Autodesk Inventor part; units mm, degrees
ref_plane "YZ Plane" through (0, 0, 0) normal (1, 0, 0) x (0, 1, 0)
ref_plane "XZ Plane" through (0, 0, 0) normal (0, 1, 0) x (-1, 0, 0)
ref_plane "XY Plane" through (0, 0, 0) normal (0, 0, 1) x (1, 0, 0)
sketch "Эскиз1" plane through (0, 0, 0) normal (0, 1, 0) x (-1, 0, 0)
  line L0 (8.9, -8.9) -> (-8.9, -8.9)
  line L1 (-8.9, -8.9) -> (-8.9, -2.1)
  line L2 (-8.9, 8.9) -> (8.9, 8.9)
  line L3 (8.9, 8.9) -> (8.9, 2.1)
  line L4 (0, 0) -> (0, -10.3494) construction
  line L5 (0, 0) -> (-17.6402, 0) construction
  circle A0 centre (10, 0) radius 0.9 construction
  circle A1 centre (-10, 0) radius 0.9 construction
  arc A2 (10, -2.1) -> (10, 2.1) centre (10, 0) ccw
  line L6 (10, -2.1) -> (8.9, -2.1)
  line L7 (10, 2.1) -> (8.9, 2.1)
  line L8 (8.9, -2.1) -> (8.9, -8.9)
  line L9 (8.9, 2.1) -> (8.9, -2.1) construction
  circle A3 centre (-10, 0) radius 0.9 construction
  arc A4 (-10, 2.1) -> (-10, -2.1) centre (-10, 0) ccw
  line L10 (-10, -2.1) -> (-8.9, -2.1)
  line L11 (-10, 2.1) -> (-8.9, 2.1)
  line L12 (-8.9, -2.1) -> (-8.9, 2.1) construction
  line L13 (-8.9, 2.1) -> (-8.9, 8.9)
  circle A5 centre (0, 0) radius 15
  arc A6 (-24.4949, -5) -> (-24.4949, 5) centre (0, 0) ccw construction
  line L14 (-14.1421, -5) -> (-27.55, -5)
  line L15 (-27.55, 5) -> (-14.1421, 5)
  arc A7 (-27.55, -5) -> (-27.55, 5) centre (0, 0) ccw construction
  arc A8 (-24.4949, 5) -> (-24.4949, -5) centre (0, 0) ccw
  arc A9 (-27.55, 5) -> (-27.55, -5) centre (0, 0) ccw
  line L16 (14.1421, -5) -> (27.55, -5)
  line L17 (27.55, 5) -> (14.1421, 5)
  arc A10 (24.4949, -5) -> (24.4949, 5) centre (0, 0) ccw
  arc A11 (27.55, -5) -> (27.55, 5) centre (0, 0) ccw
  line L18 (0, 0) -> (-17.6777, -17.6777) construction
  line L19 (0, 0) -> (25, 0) construction
  line L20 (-5, -14.1421) -> (-5, -27.55)
  line L21 (5, -27.55) -> (5, -14.1421)
  arc A12 (-5, -24.4949) -> (5, -24.4949) centre (0, 0) ccw
  arc A13 (-5, -27.55) -> (5, -27.55) centre (0, 0) ccw
  arc A14 (5, 24.4949) -> (-5, 24.4949) centre (0, 0) ccw
  line L22 (-5, 14.1421) -> (-5, 27.55)
  arc A15 (5, 27.55) -> (-5, 27.55) centre (0, 0) ccw
  line L23 (5, 27.55) -> (5, 14.1421)
  arc A16 (-13.0635, -7.3719) -> (-7.3719, -13.0635) centre (-7.0711, -7.0711) ccw
  arc A17 (7.3719, -13.0635) -> (13.0635, -7.3719) centre (7.0711, -7.0711) ccw
  arc A18 (-7.3719, 13.0635) -> (-13.0635, 7.3719) centre (-7.0711, 7.0711) ccw
  arc A19 (13.0635, 7.3719) -> (7.3719, 13.0635) centre (7.0711, 7.0711) ccw
  point P0 (17.6402, 0)
  point P1 (0, -17.6402)
  point P2 (0, 17.6402)
  point P3 (0, 25)
  point P4 (-13.0635, 7.3719)
  point P5 (-7.3719, 13.0635)
  point P6 (13.0635, -7.3719)
  point P7 (7.3719, -13.0635)
  point P8 (7.3719, 13.0635)
  point P9 (13.0635, 7.3719)
  dimension "d0" = 17.8
  dimension "d1" = 17.8
  dimension "d2" = 1.8
  dimension "d3" = 20
  dimension "d4" = 4.2
  dimension "d5" = 30
  dimension "d15" = 50
  dimension "d17" = 10
  dimension "d18" = 3
  dimension "d19" = 135
  dimension "d22" = 12
  dimension "d23" = 10
extrude "Выдавливание1" add sketch "Эскиз1" along normal blind 6 contours A5 | A5 L17 A10 L16 | A5 A19 | A17 A5 | A5 L22 A14 L23 | L21 A12 L20 A5 | A5 A18 | A16 A5 | A5 L14 A8 L15
sketch "Эскиз2" plane through (0, 0, 0) normal (0, 1, 0) x (-1, 0, 0)
  arc A0 (-13.0635, 7.3719) -> (-14.1421, 5) centre (0, 0) ccw construction
  line L0 (8.9, -2.1) -> (8.9, -8.9) construction
  line L1 (8.9, -8.9) -> (-8.9, -8.9) construction
  line L2 (-8.9, -8.9) -> (-8.9, -2.1) construction
  line L3 (-8.9, -2.1) -> (-10, -2.1) construction
  arc A1 (-10, 2.1) -> (-10, -2.1) centre (-10, 0) ccw construction
  line L4 (-10, 2.1) -> (-8.9, 2.1) construction
  line L5 (-8.9, 2.1) -> (-8.9, 8.9) construction
  line L6 (-8.9, 8.9) -> (8.9, 8.9) construction
  line L7 (8.9, 8.9) -> (8.9, 2.1) construction
  line L8 (8.9, 2.1) -> (10, 2.1) construction
  arc A2 (10, -2.1) -> (10, 2.1) centre (10, 0) ccw construction
  line L9 (10, -2.1) -> (8.9, -2.1) construction
  circle A3 centre (14.713, -5.4) radius 1.4
  line L10 (0, 0) -> (0, -15) construction
  circle A4 centre (-14.713, -5.4) radius 1.4
  arc A5 (12.5706, -3.3) -> (16.8554, -3.3) centre (14.713, -5.4) ccw
  arc A6 (-16.8554, -3.3) -> (-12.5706, -3.3) centre (-14.713, -5.4) ccw
  line L11 (14.713, -5.4) -> (14.713, -3.3) construction
  line L12 (16.8554, -3.3) -> (12.5706, -3.3)
  line L13 (-16.8554, -3.3) -> (-12.5706, -3.3)
  arc A7 (-5, 14.1421) -> (-7.3719, 13.0635) centre (0, 0) ccw
  line L14 (-5, -14.1421) -> (-5, -24.4949)
  arc A8 (-5, -24.4949) -> (5, -24.4949) centre (0, 0) ccw
  line L15 (5, -24.4949) -> (5, -14.1421)
  line L16 (14.1421, -5) -> (24.4949, -5)
  arc A9 (24.4949, -5) -> (24.4949, 5) centre (0, 0) ccw
  line L17 (24.4949, 5) -> (14.1421, 5)
  arc A10 (7.3719, 13.0635) -> (5, 14.1421) centre (0, 0) ccw
  line L18 (5, 14.1421) -> (5, 24.4949)
  arc A11 (5, 24.4949) -> (-5, 24.4949) centre (0, 0) ccw
  line L19 (-5, 24.4949) -> (-5, 14.1421)
  arc A12 (14.1421, 5) -> (13.0635, 7.3719) centre (0, 0) ccw
  line L20 (-14.1421, 5) -> (-24.4949, 5)
  arc A13 (-24.4949, 5) -> (-24.4949, -5) centre (0, 0) ccw
  line L21 (-24.4949, -5) -> (-14.1421, -5)
  arc A14 (-14.1421, -5) -> (-13.0635, -7.3719) centre (0, 0) ccw
  arc A15 (-13.0635, -7.3719) -> (-7.3719, -13.0635) centre (-7.0711, -7.0711) ccw
  arc A16 (-7.3719, -13.0635) -> (-5, -14.1421) centre (0, 0) ccw
  arc A17 (5, -14.1421) -> (7.3719, -13.0635) centre (0, 0) ccw
  arc A18 (7.3719, -13.0635) -> (13.0635, -7.3719) centre (7.0711, -7.0711) ccw
  arc A19 (13.0635, -7.3719) -> (14.1421, -5) centre (0, 0) ccw
  arc A20 (13.0635, 7.3719) -> (7.3719, 13.0635) centre (7.0711, 7.0711) ccw
  arc A21 (-7.3719, 13.0635) -> (-13.0635, 7.3719) centre (-7.0711, 7.0711) ccw
  dimension "d8" = 2.8
  dimension "d9" = 3.3
  dimension "d10" = 29.426
  dimension "d11" = 6
  dimension "d14" = 2.1
extrude "Выдавливание2" [suppressed]
extrude "Выдавливание3" add sketch "Эскиз1" along normal blind 36 contours L17 A11 L16 A10 | A14 L22 A15 L23 | L21 A13 L20 A12 | A8 L14 A9 L15
fillet "Сопряжение1" radius 2 4 edges at (0, 6, -25) (25, 6, 0) (-25, 6, 0) (0, 6, 25)
properties part number "mirror_mount_empty"
Design review of the part built by this model. Coordinates are the model's own, in mm. A direction names the side the tool comes from. Round coordinates to 2 decimals unless told otherwise and drop trailing zeros. Write each loop counter-clockwise with the first axis right and the second up, starting at its lowest first coordinate (ties: lowest second). Pieces come first, ordered by that corner, then holes.
Item 1: For pin 1 Ø1 at (y, z) = (22.5, 6.5) entering from -X; pin 2 Ø1.2 at (x, y) = (-9.5, 2) entering from +Z; pin 3 Ø0.9 at (x, y) = (9.5, 4.5) entering from -Z; pin 4 Ø6 at (y, z) = (4.5, -4.5) entering from +X, all flat-tipped, find the tip position at first contact; note any pin that passes through.
Item 2: Consider section B-B on z = 0. Give the boundary of the cut face in (x, y), and give its area (3 significant figures).
Item 3: Wall thickness on L1, parallel to X at y = 4, z = 19; L2, parallel to Z at x = -9, y = 4.5; L3, parallel to X at y = 31, z = -3: over which ranges is each line inside the solid? List them lowest first.
Item 4: Consider section A-A on y = 29. Give the boundary of the cut face in (x, z).
Item 5: Consider section D-D on z = -12. Give the boundary of the cut face in (x, y), and give its area (3 significant figures).
Item 6: Consider section C-C on z = 10. Give the boundary of the cut face in (x, y).
Item 7: For faces 4 (the cylindrical face through (25, 22, 0)), 5 (the flat face through (5, 10, -25)), 6 (the cylindrical face through (12.1, 3, 0)), list the 3-axis set-ups (+Z, -Z, +X, -X, +Y, -Y) from which the entire face can be reached by the end or side of a thin tool; tool diameter is ignored.
Item 8: Draft analysis for pull direction Z (two halves, no side actions). For faces 1 (the cylindrical face through (-13.662, 2.958, -6.193)), 2 (the cylindrical face through (0, 22, 25)), 3 (the flat face through (5, 10, 25)), state which applies: released by +Z, released by -Z, zero draft, split by the parting line, or undercut.
Check values:
1. pin 1: passes through
1. pin 2: stops at z = 12.79
1. pin 3: stops at z = -12.74
1. pin 4: stops at x = 27.96
2. outline: (-28, 0) - (-12.1, 0) - (-12.1, 6) - (-23, 6) arc R2 cw to (-25, 8) - (-25, 36) - (-28, 36) - close; (12.1, 0) - (28, 0) - (28, 36) - (25, 36) - (25, 8) arc R2 cw to (23, 6) - (12.1, 6) - close
2. area: 373 mm2
3. L1: x = -5 to 5
3. L2: z = -12.75 to -2.1, 2.1 to 12.75
3. L3: x = -27.84 to -24.82, 24.82 to 27.84
4. outline: (-27.55, -5) - (-24.49, -5) arc R25 cw to (-24.49, 5) - (-27.55, 5) arc R28 ccw to start; (-5, -27.55) arc R28 ccw to (5, -27.55) - (5, -24.49) arc R25 cw to (-5, -24.49) - close; (-5, 24.49) arc R25 cw to (5, 24.49) - (5, 27.55) arc R28 ccw to (-5, 27.55) - close; (24.49, -5) - (27.55, -5) arc R28 ccw to (27.55, 5) - (24.49, 5) arc R25 cw to start
5. outline: (-10.49, 0) - (10.49, 0) - (10.49, 6) - (-10.49, 6) - close
5. area: 126 mm2
6. outline: (-12.31, 0) - (12.31, 0) - (12.31, 6) - (-12.31, 6) - close
7. face 4: +Y
7. face 5: -Z, +X, +Y, -Y
7. face 6: +Y, -Y
8. face 1: released by -Z
8. face 2: undercut
8. face 3: zero draft
